Could you check a few things on this model? Use its own coordinates, in mm. A direction names the side the tool comes from. Coordinates: 2 decimals unless noted, no trailing zeros. Order: outer loops, then holes, each group sorted by start corner. A loop starts at its lowest first (then second) coordinate and runs counter-clockwise, first axis right, second up. Notation, with made-up numbers: M -15,46.25 L 10,46.25 A24 ccw 10,80.25 Z; hole C 53,63 d7. An arc over 180 degrees is marked long. Write item = value, one per line. Start each with the question number.
from build123d import *

# Parameters (mm, degrees)
SKETCH_2_W             = 64.02174429
SKETCH_2_H             = 9.248919907
CUT_EXTRUDE_1_DEPTH    = 49
HOLE_WIZARD_M4_2_D     = 3.3
HOLE_WIZARD_M4_2_DEPTH = 5.5
HOLE_WIZARD_M4_2_TIP   = 0.991420021
HOLE_WIZARD_M6_2_D     = 5
HOLE_WIZARD_M6_2_DEPTH = 5.5
HOLE_WIZARD_M6_2_TIP   = 1.502151548


with BuildPart() as part:
    # 草图1 → 旋转1 (revolve)
    with BuildSketch(Plane(origin=(0, 0, 0), x_dir=(1, 0, 0), z_dir=(0, 1, 0)), mode=Mode.PRIVATE) as revolve_1_sk:
        Polygon((22.5, 7.5), (22.5, -7.5), (13.75, -7.5), (13.75, -3), (14.35, -3), (14.35, -2), (12, -2), (12, 2), (14.35, 2), (14.35, 3), (13.75, 3), (13.75, 7.5), align=None)
    revolve(revolve_1_sk.sketch.rotate(Axis((0, 0, -31.9390681), (0, 0, 1)), 180), axis=Axis((0, 0, -31.9390681), (0, 0, 1)))  # turned: the seam where the file's is

    # 草图2 → 切除-拉伸1 (cut)
    with BuildSketch(Plane.XY.offset(7.5)):
        with Locations((-1.141100508, 26.124459954)):
            Rectangle(SKETCH_2_W, SKETCH_2_H)
        with Locations((-1.141100508, -26.124459954)):
            Rectangle(SKETCH_2_W, SKETCH_2_H)
    extrude(amount=-CUT_EXTRUDE_1_DEPTH, mode=Mode.SUBTRACT)

    # M4 螺纹孔2
    with Locations(Plane(origin=(0, 21.5, 0), x_dir=(1, 0, 0), z_dir=(0, 1, 0))):
        with Locations((0, 0)):
            Hole(HOLE_WIZARD_M4_2_D / 2, depth=HOLE_WIZARD_M4_2_DEPTH)
            with Locations((0, 0, -(HOLE_WIZARD_M4_2_DEPTH + HOLE_WIZARD_M4_2_TIP / 2))):  # 118° drill point
                Cone(0, HOLE_WIZARD_M4_2_D / 2, HOLE_WIZARD_M4_2_TIP, mode=Mode.SUBTRACT)

    # M6 螺纹孔2
    with Locations(Plane(origin=(0, -21.5, 0), x_dir=(-1, 0, 0), z_dir=(0, -1, 0))):
        with Locations((0, 0)):
            Hole(HOLE_WIZARD_M6_2_D / 2, depth=HOLE_WIZARD_M6_2_DEPTH)
            with Locations((0, 0, -(HOLE_WIZARD_M6_2_DEPTH + HOLE_WIZARD_M6_2_TIP / 2))):  # 118° drill point
                Cone(0, HOLE_WIZARD_M6_2_D / 2, HOLE_WIZARD_M6_2_TIP, mode=Mode.SUBTRACT)


solid = part.part
(1) Imagine slicing it at B-B on z = 5. List the corners of the cut face in (x, y) for me.
(2) Imagine slicing it at D-D on x = 16. List the corners of the cut face in (y, z) for me.
(3) For faces 4 (the cylindrical face through (-6.34, 12.2, 5.22)), 5 (the cylindrical face through (-6.34, 12.2, -5.28)), 6 (the flat face through (3, 12, 2)), which set-ups out of +Z, -Z, +X, -X, +Y, -Y let a thin tool reach every point of the face, with its end or its side?
(4) Thinking about a two-plate mould opening in Y: for faces 1 (the cylindrical face through (22.496, -0.401, 0.105)), 2 (the flat face through (3, -21.5, 0)), 3 (the flat face through (-3, 12, -2)), which applies, released by +Y, released by -Y, zero draft, split by the parting line, or undercut?
(5) Imagine slicing it at A-A on y = -9. List the corners of the cut face in (x, z) for me, plus the area to 3 significant figures.
(6) Imagine slicing it at C-C on y = 0. List the corners of the cut face in (x, z) for me.
(7) Will these pins go through, and if not, where does the flat tip stop? P1, Ø3, axis at x = 0, z = 0, coming from the +Y side; P2, Ø1, axis at x = -18, y = -15.5, coming from the -Z side; P3, Ø6, axis at x = -14.5, z = -4, coming from the -Y side; P4, Ø1, axis at x = 14.5, z = -2, coming from the +Y side.
(8) Please list where these lines run through material, in increasing order: probe 1 along Z at (x, y) = (0, -18.35); probe 2 along Z at (x, y) = (0, 19); probe 3 along Y at (x, z) = (0, 4.4). Write a range as from..to.
Response:
q1.outline = M -6.63,-21.5 L 6.63,-21.5 A22.5 ccw 6.63,21.5 L -6.63,21.5 A22.5 ccw Z; hole C 0,0 d27.5
q2.outline = M -15.82,-7.5 L 15.82,-7.5 L 15.82,7.5 L -15.82,7.5 Z
q3.face_4 = +Z
q3.face_5 = -Z
q3.face_6 = none
q4.face_1 = split by the parting line
q4.face_2 = released by -Y
q4.face_3 = undercut
q5.outline = M -20.62,-7.5 L -10.4,-7.5 L -10.4,-3 L -11.18,-3 L -11.18,-2 L -7.94,-2 L -7.94,2 L -11.18,2 L -11.18,3 L -10.4,3 L -10.4,7.5 L -20.62,7.5 Z; M 7.94,-2 L 11.18,-2 L 11.18,-3 L 10.4,-3 L 10.4,-7.5 L 20.62,-7.5 L 20.62,7.5 L 10.4,7.5 L 10.4,3 L 11.18,3 L 11.18,2 L 7.94,2 Z
q5.area = 323 mm2
q6.outline = M -22.5,-7.5 L -13.75,-7.5 L -13.75,-3 L -14.35,-3 L -14.35,-2 L -12,-2 L -12,2 L -14.35,2 L -14.35,3 L -13.75,3 L -13.75,7.5 L -22.5,7.5 Z; M 12,-2 L 14.35,-2 L 14.35,-3 L 13.75,-3 L 13.75,-7.5 L 22.5,-7.5 L 22.5,7.5 L 13.75,7.5 L 13.75,3 L 14.35,3 L 14.35,2 L 12,2 Z
q7.P1 = 15.91
q7.P2 = through
q7.P3 = -19.34
q7.P4 = 17.61
q8.probe_1 = -7.5..-2.5, 2.5..7.5
q8.probe_2 = -7.5..-1.65, 1.65..7.5
q8.probe_3 = -21.5..-13.75, 13.75..21.5
